from build123d import *

# Parameters (mm, degrees)
F1_DEPTH  = 20
F2_R      = 1.75
F3_DEPTH  = 3
F6_W      = 16
F6_H      = 35.2884006159
F7_DEPTH  = 12.5
F8_R      = 3
F10_DEPTH = 25


with BuildPart() as f1:
    # F0 (on Right) → F1 (new body)
    with BuildSketch(Plane.YZ):
        with BuildLine():
            ThreePointArc((-4.1024079025, -2.8327919807), (-4.4198799521, -1.3762495526), (-5.3147026709, -0.1839422731))
            Line((-5.3147026709, -0.1839422731), (-7.5675635352, 0.6670345679))
            ThreePointArc((-7.5675635352, 0.6670345679), (-10.0649314774, -0.3456294121), (-11.1024079025, -2.8327919807))
            Line((-11.1024079025, -2.8327919807), (-7.6024079025, -2.8327919807))
            Line((-7.6024079025, -2.8327919807), (-4.1024079025, -2.8327919807))
        make_face()
        with BuildLine():
            Line((-10.9565098687, -3.8327919807), (-7.6024079025, -3.8327919807))
            Line((-7.6024079025, -3.8327919807), (-7.6024079025, -2.8327919807))
            Line((-7.6024079025, -2.8327919807), (-11.1024079025, -2.8327919807))
            ThreePointArc((-11.1024079025, -2.8327919807), (-11.0657413316, -3.3380855182), (-10.9565098687, -3.8327919807))
        make_face()
        with BuildLine():
            Line((-7.6024079025, -3.8327919807), (-4.2483059362, -3.8327919807))
            ThreePointArc((-4.2483059362, -3.8327919807), (-4.1390744734, -3.3380855182), (-4.1024079025, -2.8327919807))
            Line((-4.1024079025, -2.8327919807), (-7.6024079025, -2.8327919807))
            Line((-7.6024079025, -2.8327919807), (-7.6024079025, -3.8327919807))
        make_face()
        with BuildLine():
            Line((-7.6024079025, -6.3327919807), (-7.6024079025, -3.8327919807))
            Line((-7.6024079025, -3.8327919807), (-10.9565098687, -3.8327919807))
            ThreePointArc((-10.9565098687, -3.8327919807), (-9.6940579688, -5.6390350208), (-7.6024079025, -6.3327919807))
        make_face()
        with BuildLine():
            ThreePointArc((-7.6024079025, -6.3327919807), (-5.5107578361, -5.6390350208), (-4.2483059362, -3.8327919807))
            Line((-4.2483059362, -3.8327919807), (-7.6024079025, -3.8327919807))
            Line((-7.6024079025, -3.8327919807), (-7.6024079025, -6.3327919807))
        make_face()
        with BuildLine():
            Line((14.8975920975, -3.8327919807), (4.3451967649, -3.8327919807))
            Line((4.3451967649, -3.8327919807), (-4.2483059362, -3.8327919807))
            ThreePointArc((-4.2483059362, -3.8327919807), (-5.5107578361, -5.6390350208), (-7.6024079025, -6.3327919807))
            Line((-7.6024079025, -6.3327919807), (14.8975920975, -6.3327919807))
            Line((14.8975920975, -6.3327919807), (14.8975920975, -3.8327919807))
        make_face()
        with BuildLine():
            Line((-4.2483059362, -3.8327919807), (4.3451967649, -3.8327919807))
            Line((4.3451967649, -3.8327919807), (-5.3147026709, -0.1839422731))
            ThreePointArc((-5.3147026709, -0.1839422731), (-4.4198799521, -1.3762495526), (-4.1024079025, -2.8327919807))
            ThreePointArc((-4.1024079025, -2.8327919807), (-4.1390744734, -3.3380855182), (-4.2483059362, -3.8327919807))
        make_face()
    extrude(amount=F1_DEPTH)



with BuildPart() as f3:
    # F2 (on face) → F3 (new body)
    with BuildSketch(Plane(origin=(0, 0, 0), x_dir=(0, -1, 0), z_dir=(-1, 0, 0))):
        with Locations((7.6024079025, -2.8327919807)):
            Circle(F2_R)
    extrude(amount=F3_DEPTH)


with BuildPart() as f1_1:
    add(f1.part)

    add(f3.part)  # F5 merges F3
    # F5: F3 across plane
    add(f3.part.mirror(Plane.YZ.offset(10)))

    # F6 (on face) → F7 (cut, symmetric)
    with BuildSketch(Plane.XY.offset(-3.8327919807)):
        with Locations((10, -13.2466082104)):
            Rectangle(F6_W, F6_H)
    extrude(amount=F7_DEPTH, both=True, mode=Mode.SUBTRACT)

    # F8
    f8_edges = [f1_1.edges().sort_by_distance(p)[0] for p in [
        (20, 14.897592, -5.082792),
        (0, 14.897592, -5.082792),
    ]]
    fillet(f8_edges, radius=F8_R)


with BuildPart() as f10:
    # F9 (on Front) → F10 (new body)
    with BuildSketch(Plane.XZ):
        Polygon((20.3534542639, 3.3057429828), (20.3534542639, 0.1906278993), (23.9095985889, -4.0474198759), (23.9095985889, 7.1602235548), (-3.9095985889, 7.1602235548), (-3.9095985889, -4.0474198759), (-0.3534542639, 0.1906278993), (-0.3534542639, 3.3057429828), align=None)
    extrude(amount=F10_DEPTH)


with BuildPart() as f1_2:
    add(f1_1.part)

    # F11: cut F10
    add(f10.part, mode=Mode.SUBTRACT)


solid = f1_2.part
The model under review builds one solid part; all positions refer to its coordinate system, in mm. A direction names the side the tool comes from. Round coordinates to 2 decimals unless told otherwise and drop trailing zeros. Loops run counter-clockwise (first coordinate to the right, second up) from the corner with the lowest first, then second, coordinate; pieces in that order, holes last. Notation, with made-up numbers: (29, 23) -> (50, 23) arc R31 cw to (50, 51) -> close; hole circle Ø8 at (63, 86). An arc over 180 degrees is marked (long way). Write item = value, one per line. Start each with the question number.
Item 1: Insertion check: pin 1 (1.5 mm diameter, centred on x = 0, y = -0.5, fed in from +Z); pin 2 (4 mm diameter, centred on y = 2, z = -4, fed in from -X); pin 3 (1 mm diameter, centred on x = 5, y = 10, fed in from +Z). Each pin has a flat end and moves straight along its axis. Give the tip position at first contact, or say it passes through.
Item 2: To check wall thickness, follow L1, parallel to X at y = -8.5, z = -0.5; L2, parallel to Z at x = 5, y = 11; L3, parallel to Y at x = 3.5, z = -5. State the ranges of each line that lie inside material, in increasing order.
Item 3: Take a section at A-A on y = -3.75. Give the boundary of the cut face in (x, z), plus the area to 3 significant figures.
Item 4: Take a section at D-D on y = 11.5. Give the boundary of the cut face in (x, z), plus the area to 3 significant figures.
Item 5: Take a section at B-B on z = -2.5. Give the boundary of the cut face in (x, y).
Item 6: For faces 1 (the flat face through (2, -5, -4)), 2 (the flat face through (10, 10, -3.833)), 3 (the cylindrical face through (-1.15, -7.22, -4.54)), list the 3-axis set-ups (+Z, -Z, +X, -X, +Y, -Y) from which the entire face can be reached by the end or side of a thin tool; tool diameter is ignored.
Item 7: Take a section at C-C on y = 0. Give the boundary of the cut face in (x, z).
Result:
q1.pin_1 = -1.72
q1.pin_2 = 0
q1.pin_3 = -3.83
q2.L1 = 0 to 2, 18 to 20
q2.L2 = -6.33 to -3.83
q2.L3 = 4.4 to 14.9
q3.outline = (0, -6.33) -> (2, -6.33) -> (2, -0.77) -> (0, -0.77) -> close; (18, -6.33) -> (20, -6.33) -> (20, -0.77) -> (18, -0.77) -> close
q3.area = 22.2 mm²
q4.outline = (0, -6.33) -> (20, -6.33) -> (20, -3.83) -> (0, -3.83) -> close
q4.area = 50.0 mm²
q5.outline = (-2.61, -9.32) -> (0, -9.32) -> (0, -11.09) -> (2, -11.09) -> (2, 0.82) -> (0, 0.82) -> (0, -5.88) -> (-2.61, -5.88) -> close; (18, -11.09) -> (20, -11.09) -> (20, -9.32) -> (22.61, -9.32) -> (22.61, -5.88) -> (20, -5.88) -> (20, 0.82) -> (18, 0.82) -> close
q6.face_1 = +Z, -Z, -Y
q6.face_2 = +Z, +X, -X, +Y
q6.face_3 = -X
q7.outline = (0, -6.33) -> (2, -6.33) -> (2, -2.19) -> (0, -2.19) -> close; (18, -6.33) -> (20, -6.33) -> (20, -2.19) -> (18, -2.19) -> close
